Autodesk Inventor part; units mm, degrees
ref_plane "YZ Plane" through (0, 0, 0) normal (1, 0, 0) x (0, 1, 0)
ref_plane "XZ Plane" through (0, 0, 0) normal (0, 1, 0) x (-1, 0, 0)
ref_plane "XY Plane" through (0, 0, 0) normal (0, 0, 1) x (1, 0, 0)
sketch "Sketch1" plane through (0, 0, 0) normal (0, 0, 1) x (1, 0, 0)
  circle A0 centre (0, 0) radius 18
  dimension "d0" = 36
extrude "Extrusion1" add sketch "Sketch1" along normal blind 6
sketch "Sketch2" plane through (0, 0, 6) normal (0, 0, 1) x (1, 0, 0)
  circle A0 centre (0, 0) radius 16
  dimension "d3" = 32
extrude "Extrusion2" add sketch "Sketch2" along normal blind 6
sketch "Sketch3" plane through (0, 0, 12) normal (0, 0, 1) x (1, 0, 0)
  circle A0 centre (0, 0) radius 7
  circle A1 centre (-8.4853, 8.4853) radius 2
  circle A2 centre (-12, 0) radius 2
  circle A3 centre (-8.4853, -8.4853) radius 2
  circle A4 centre (0, -12) radius 2
  line L0 (-8.4853, 8.4853) -> (0, 0) construction
  line L1 (-7, 0) -> (0, 0) construction
  circle A5 centre (8.4853, -8.4853) radius 2
  circle A6 centre (12, 0) radius 2
  circle A7 centre (8.4853, 8.4853) radius 2
  circle A8 centre (0, 12) radius 2
  dimension "d6" = 14
  dimension "d7" = 4
  dimension "d12" = 360
  dimension "d16" = 45
  dimension "d17" = 12
extrude "Extrusion3" cut sketch "Sketch3" against normal through all
properties part number "SecondStageArmClamp" material "PC/ABS Plastic"
Check sheet for the modelled part. Datum: model origin and axes. Units: mm. A direction names the side the tool comes from. Round coordinates to 2 decimals unless told otherwise and drop trailing zeros. Loops run counter-clockwise (first coordinate to the right, second up) from the corner with the lowest first, then second, coordinate; pieces in that order, holes last. Notation, with made-up numbers: (67, 67.25) - (107, 67.25) arc R33 ccw to (107, 100.25) - close; hole circle Ø6 at (2, -13.75). An arc over 180 degrees is marked (long way). Answer as CSV lines item,"result". Start each with the question number.
Item 1: Section check B-B (y = 12). Record the boundary of the cut face in (x, z), and give its area (3 significant figures).
Item 2: Section check C-C (x = 13.5). Record the boundary of the cut face in (y, z), and give its area (3 significant figures).
Item 3: Set-up check for faces 4 (the cylindrical face through (10.333, -9.251, 6.084)), 5 (the cylindrical face through (-3.47, 15.62, 8.96)): record each of +Z, -Z, +X, -X, +Y, -Y from which the full face is reachable in a straight line by a thin tool's end or side.
Item 4: Section check A-A (x = 0). Record the boundary of the cut face in (y, z).
Item 5: Release check for a two-part mould opening along Y. For faces 1 (the flat face through (0, -8, 0)), 2 (the cylindrical face through (-2.343, -17.847, 2.958)), 3 (the cylindrical face through (-6.58, -7.88, 6.08)) record: +Y half, -Y half, draft (parallel to the pull), parting line (faces both ways), or undercut.
Item 6: Depth check by flat-ended pin: P1, Ø3, axis at y = 9, z = 10.5, coming from the +X side; P2, Ø6, axis at x = -4, z = 10, coming from the -Y side; P3, Ø3, axis at y = 13, z = 8.5, coming from the +X side. Enter the tip coordinate at first touch or a pass-through.
Item 7: Section check D-D (x = -9). Record the boundary of the cut face in (y, z).
Item 8: Scan lines: line 1 (Y direction, x = 0, z = 6.5); line 2 (Y direction, x = -1, z = 5); line 3 (X direction, y = 8, z = 7.5). Record each from-to range of solid material in increasing order. Write a range as [from, to].
Report:
1,outline,"(-13.42, 0) - (-2, 0) - (-2, 12) - (-10.58, 12) - (-10.58, 6) - (-13.42, 6) - close; (2, 0) - (13.42, 0) - (13.42, 6) - (10.58, 6) - (10.58, 12) - (2, 12) - close"
1,area,"240 mm2"
2,outline,"(-11.91, 0) - (-1.32, 0) - (-1.32, 12) - (-8.59, 12) - (-8.59, 6) - (-11.91, 6) - close; (1.32, 0) - (11.91, 0) - (11.91, 6) - (8.59, 6) - (8.59, 12) - (1.32, 12) - close"
2,area,"214 mm2"
3,face 4,"+Z, -Z"
3,face 5,"+Z"
4,outline,"(-18, 0) - (-14, 0) - (-14, 12) - (-16, 12) - (-16, 6) - (-18, 6) - close; (-10, 0) - (-7, 0) - (-7, 12) - (-10, 12) - close; (7, 0) - (10, 0) - (10, 12) - (7, 12) - close; (14, 0) - (18, 0) - (18, 6) - (16, 6) - (16, 12) - (14, 12) - close"
5,face 1,"draft"
5,face 2,"parting line"
5,face 3,"undercut"
6,P1,"stops at x = 14.13"
6,P2,"stops at y = -15.97"
6,P3,"stops at x = 11.12"
7,outline,"(-15.59, 0) - (-10.42, 0) - (-10.42, 12) - (-13.23, 12) - (-13.23, 6) - (-15.59, 6) - close; (-6.55, 0) - (6.55, 0) - (6.55, 12) - (-6.55, 12) - close; (10.42, 0) - (15.59, 0) - (15.59, 6) - (13.23, 6) - (13.23, 12) - (10.42, 12) - close"
8,line 1,"y = [-16, -14], [-10, -7], [7, 10], [14, 16]"
8,line 2,"y = [-17.97, -13.73], [-10.27, -6.93], [6.93, 10.27], [13.73, 17.97]"
8,line 3,"x = [-13.86, -10.43], [-6.55, 6.55], [10.43, 13.86]"
